from build123d import *

# Parameters (mm, degrees)
FASE1_SIZE = 0.5
FASE2_SIZE = 0.5


with BuildPart() as part:
    # Skizze1 → Rotation1 (revolve)
    with BuildSketch(Plane.XY, mode=Mode.PRIVATE) as rotation1_sk:
        Polygon((2, 0), (2, -6), (5.95, -6), (5.95, -5), (3.95, -5), (3.95, 0), align=None)
    revolve(rotation1_sk.sketch.rotate(Axis((0, 16.559935445, 0), (0, -1, 0)), 90), axis=Axis((0, 16.559935445, 0), (0, -1, 0)))

    # Fase1
    fase1_edges = [part.edges().sort_by_distance(p)[0] for p in [
        (0, 0, -3.95),
    ]]
    chamfer(fase1_edges, length=FASE1_SIZE)

    # Fase2
    fase2_edges = [part.edges().sort_by_distance(p)[0] for p in [
        (0, -6, -2),
    ]]
    chamfer(fase2_edges, length=FASE2_SIZE)


solid = part.part
The listing builds one solid part. Answer for the finished solid, in the listing's coordinates (mm). Coordinates: 2 decimals unless noted, no trailing zeros. Write each loop counter-clockwise with the first axis right and the second up, starting at its lowest first coordinate (ties: lowest second). Pieces come first, ordered by that corner, then holes. Notation, with made-up numbers: M -5.5,-38.5 L 19.5,-38.5 A11 cw 19.5,-31.5 Z; hole C 20,-36.75 d8. An arc over 180 degrees is marked long. Use one line per item in the form item = value.
Item 1: Find section A-A, the plane z = 0. Give the vertices of the cut face in (x, y).
Model answer:
outline = M -5.95,-6 L -2.5,-6 L -2,-5.5 L -2,0 L -3.45,0 L -3.95,-0.5 L -3.95,-5 L -5.95,-5 Z; M 2,-5.5 L 2.5,-6 L 5.95,-6 L 5.95,-5 L 3.95,-5 L 3.95,-0.5 L 3.45,0 L 2,0 Z
Item 2: Find section D-D, the plane z = -4.5. Give the vertices of the cut face in (x, y), plus the area to 3 significant figures.
Model answer:
outline = M -3.89,-6 L 3.89,-6 L 3.89,-5 L -3.89,-5 Z
area = 7.79 mm2
Item 3: The mould has two halves that part along Z. Classify faces 1 (the face through (-2.67, -2.72, -2.91)), 2 (the face through (2, -3, 0)), 3 (the face through (1, -5, 4)): released by +Z, released by -Z, zero draft, split by the parting line, or undercut.
Model answer:
face_1 = split by the parting line
face_2 = undercut
face_3 = zero draft
Item 4: Find section C-C, the plane y = -4. Give the vertices of the cut face in (x, z), plus the area to 3 significant figures.
Model answer:
outline = C 0,0 d7.9; hole C 0,0 d4
area = 36.5 mm2
Item 5: Given P1, Ø3, axis at x = -3.5, y = -4, coming from the -Z side; P2, Ø3, axis at x = 3.5, y = -3, coming from the -Z side; P3, Ø1.5, axis at x = -4, z = 3, coming from the +Y side, each flat-ended and moving along its own axis, determine where each tip first touches the part or whether it passes through.
Model answer:
P1 = -5.45
P2 = -3.41
P3 = -5
Item 6: Find the intervals of material crossed by probe 1 along X at (y, z) = (-1.95, 0); probe 2 along Y at (x, z) = (5, 1.75); probe 3 along X at (y, z) = (-4.65, -1.5), in increasing order.
Model answer:
probe_1 = -3.95 to -2, 2 to 3.95
probe_2 = -6 to -5
probe_3 = -3.65 to -1.32, 1.32 to 3.65
Item 7: Find section B-B, the plane x = 0. Give the vertices of the cut face in (y, z).
Model answer:
outline = M -6,-5.95 L -5,-5.95 L -5,-3.95 L -0.5,-3.95 L 0,-3.45 L 0,-2 L -5.5,-2 L -6,-2.5 Z; M -6,2.5 L -5.5,2 L 0,2 L 0,3.45 L -0.5,3.95 L -5,3.95 L -5,5.95 L -6,5.95 Z
